Verification items for the finished model (mm, model axes). Coordinates: 2 decimals unless noted, no trailing zeros. Order: outer loops, then holes, each group sorted by start corner. A loop starts at its lowest first (then second) coordinate and runs counter-clockwise, first axis right, second up. Notation, with made-up numbers: (12, -13) -> (16, -13) arc R9 cw to (16, -9) -> close; hole circle Ø2 at (-32, 73.25). An arc over 180 degrees is marked (long way). Use CSV: the item, a comma, the result in double quotes. Start each with the question number.
1) Sectioned sample at A-A on y = -142.5. Record the boundary of the cut face in (x, z).
2) Go/stop test with flat-tipped pins: pin 1 (12 mm diameter, centred on x = -8.5, z = 1.5, fed in from +Y); pin 2 (1 mm diameter, centred on x = -11, y = -165, fed in from +Z); pin 3 (8 mm diameter, centred on x = -4, y = -267.5, fed in from -Z); pin 4 (10 mm diameter, centred on y = -234, z = 6.5, fed in from +X). Record where each tip stops, or that it passes through.
3) Scan lines: line 1 along Z through (x, y) = (-1, -208); line 2 along Z through (x, y) = (-19, -133); line 3 along X through (y, z) = (-252, 1.5). Record each from-to range of solid material in increasing order.
from build123d import *

# Parameters (mm, degrees)
F0_R     = 24.9
F1_DEPTH = 300
F2_SIZE  = 2
F3_SIZE  = 2


with BuildPart() as f1:
    # F0 (on Front) → F1 (new body)
    with BuildSketch(Plane.XZ):
        Circle(F0_R)
    extrude(amount=F1_DEPTH)

    # F2
    f2_edges = [f1.edges().sort_by_distance(p)[0] for p in [
        (-24.9, -300, 0),
    ]]
    chamfer(f2_edges, length=F2_SIZE)

    # F3
    f3_edges = [f1.edges().sort_by_distance(p)[0] for p in [
        (-24.9, 0, 0),
    ]]
    chamfer(f3_edges, length=F3_SIZE)


solid = f1.part
Answers follow:
1,outline,"circle Ø49.8 at (0, 0)"
2,pin 1,"stops at y = 0"
2,pin 2,"stops at z = 22.58"
2,pin 3,"stops at z = -24.9"
2,pin 4,"stops at x = 24.85"
3,line 1,"z = -24.88 to 24.88"
3,line 2,"z = -16.09 to 16.09"
3,line 3,"x = -24.85 to 24.85"
